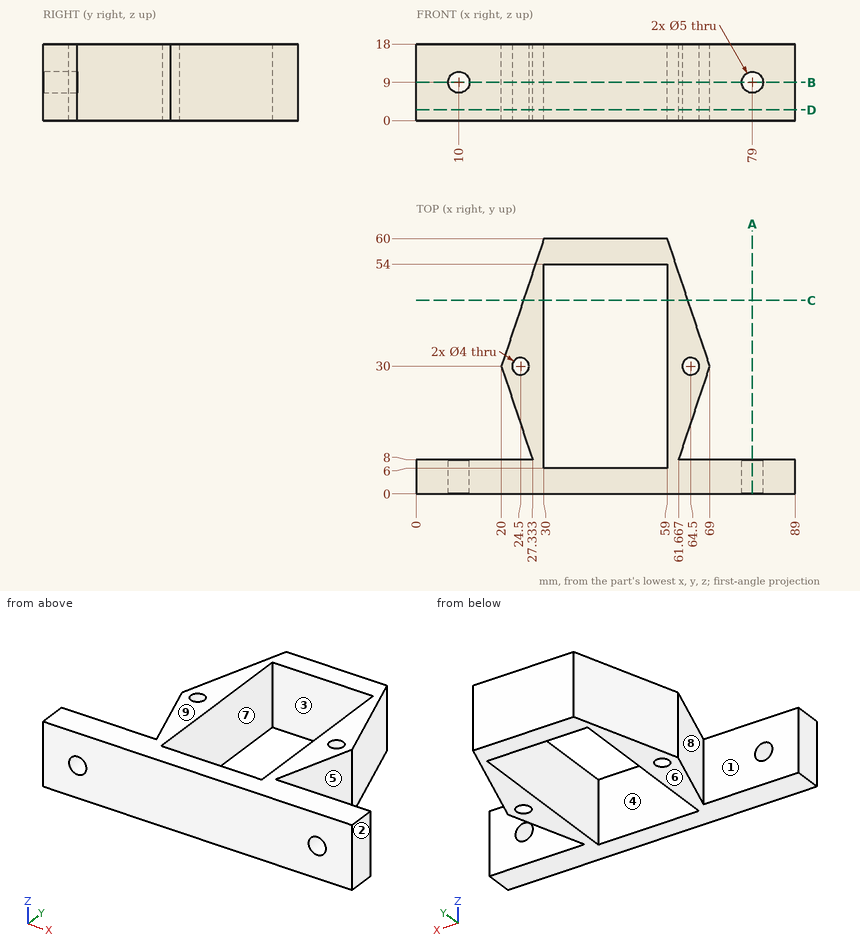
Could you check a few things on this drawing? It's one solid part, dimensions in mm from its lowest x, y, z. A direction names the side the tool comes from. Give positions to 0.01 mm unless a question says otherwise; leave off trailing zeros. Loops run counter-clockwise (first coordinate to the right, second up) from the corner with the lowest first, then second, coordinate; pieces in that order, holes last. Notation, with made-up numbers: M -10,-30.75 L -5,-30.75 A22 ccw -5,-8.75 Z; hole C -4.75,21.5 d10. An arc over 180 degrees is marked long. Answer as a JSON object with one key per item and string values.
Q1. For the marked faces 5, 6, 7, 8 and 9, which set-ups out of +Z, -Z, +X, -X, +Y, -Y let a thin tool reach every point of the face, with its end or its side?
Values found:
{"face 5": "+Z, -Z, +X", "face 6": "-Z, +X, -X, +Y, -Y", "face 7": "+Z, -Z", "face 8": "+Z, -Z, -X", "face 9": "+Z, +X, -X, +Y, -Y"}
Q2. Suppose I cut it at B-B, the plane z = 9. List the corners of the cut face in (x, y) for me, plus the area to 3 significant figures.
Values found:
{"outline": "M 0,0 L 7.5,0 L 7.5,8 L 0,8 Z; M 12.5,0 L 76.5,0 L 76.5,8 L 61.67,8 L 69,30 L 59,60 L 30,60 L 20,30 L 27.33,8 L 12.5,8 Z; M 81.5,0 L 89,0 L 89,8 L 81.5,8 Z; hole C 24.5,30 d4; hole M 30,6 L 59,6 L 59,54 L 30,54 Z; hole C 64.5,30 d4", "area": "1,300 mm²"}
Q3. Suppose I cut it at A-A, the plane x = 79. List the corners of the cut face in (y, z) for me.
Values found:
{"outline": "M 0,0 L 8,0 L 8,6.5 L 0,6.5 Z; M 0,11.5 L 8,11.5 L 8,18 L 0,18 Z"}
Q4. Suppose I cut it at C-C, the plane y = 45.5. List the corners of the cut face in (x, z) for me, plus the area to 3 significant figures.
Values found:
{"outline": "M 25.17,0 L 30,0 L 30,18 L 25.17,18 Z; M 59,0 L 63.83,0 L 63.83,18 L 59,18 Z", "area": "174 mm²"}
Q5. If we mould it in two halves opening along X, with no side actions, what happens to the marked faces 1, 2, 3 and 4? For each: pulls with the +X half, pulls with the -X half, needs draft (parallel to the pull), parting line crosses it, or undercut.
Values found:
{"face 1": "needs draft", "face 2": "pulls with the +X half", "face 3": "undercut", "face 4": "undercut"}
Q6. If I drill on probe 1 along X at (y, z) = (5, 9); probe 2 along X at (y, z) = (6.25, 9); probe 3 along Z at (x, y) = (79, 5.25), over which ranges is the centre line in solid material (lowest first)? Write a range as [from, to].
Values found:
{"probe 1": "x = [0, 7.5], [12.5, 76.5], [81.5, 89]", "probe 2": "x = [0, 7.5], [12.5, 30], [59, 76.5], [81.5, 89]", "probe 3": "z = [0, 6.5], [11.5, 18]"}
Q7. Suppose I cut it at D-D, the plane z = 2.5. List the corners of the cut face in (x, y) for me, plus the area to 3 significant figures.
Values found:
{"outline": "M 0,0 L 89,0 L 89,8 L 61.67,8 L 69,30 L 59,60 L 30,60 L 20,30 L 27.33,8 L 0,8 Z; hole C 24.5,30 d4; hole M 30,6 L 59,6 L 59,54 L 30,54 Z; hole C 64.5,30 d4", "area": "1,380 mm²"}
Q8. For P1, Ø9, axis at y = 35.5, z = 10, coming from the -X side; P2, Ø6, axis at x = 16, y = 30, coming from the -Z side; P3, Ø8, axis at x = 10, z = 9, coming from the +Y side; P4, Ø4, axis at y = 43.5, z = 6.5, coming from the +X side, each with a flat end and sliding along its axis, tell me the tip position at first contact or that it passes through.
Values found:
{"P1": "stops at x = 20.33", "P2": "passes through", "P3": "stops at y = 8", "P4": "stops at x = 65.17"}
